For this review, take the finished solid that the model builds, in its own axes (mm). A direction names the side the tool comes from. Coordinates: 2 decimals unless noted, no trailing zeros. Loops run counter-clockwise (first coordinate to the right, second up) from the corner with the lowest first, then second, coordinate; pieces in that order, holes last. Notation, with made-up numbers: M 67,30 L 98,30 A23 ccw 98,41 Z; hole C -17.75,-13.5 d7. An arc over 180 degrees is marked long. Answer as a JSON object with one key per item and string values. Group by question number.
Item 1: Tool access review of faces 1 (the face through (0, 3, 1.85)), 2 (the face through (0, 3, -1.85)), 3 (the face through (-1.595, 3.161, -0.938)), 4 (the face through (-0.05, 6, -2.04)): name each direction out of +Z, -Z, +X, -X, +Y, -Y from which nothing blocks a thin tool from reaching the whole face with its end or side.
Item 2: Add section D-D (y = 6.5). State the section outline as (x, z) points.
Item 3: Wall thickness on L1, parallel to Y at x = -2, z = -2; L2, parallel to Z at x = 0.75, y = 3.5: over which ranges is each line inside the solid? List them lowest first. Write a range as from..to.
Item 4: Add section B-B (x = -0.5). State the section outline as (y, z) points.
Item 5: Insertion check: pin 1 (2 mm diameter, centred on x = 1.5, y = 4.5, fed in from -Z); pin 2 (2.5 mm diameter, centred on x = 0, y = 4, fed in from +Z). Each pin has a flat end and moves straight along its axis. Give the tip position at first contact, or say it passes through.
Item 6: Add section C-C (z = 1.25). State the section outline as (x, y) points.
Item 7: Add section A-A (y = 2.75). State the section outline as (x, z) points, then the cut area to 3 significant figures.
from build123d import *

# Parameters (mm, degrees)
BOSS_EXTRUDE1_DEPTH = 6
BOSS_EXTRUDE2_DEPTH = 1.2
CHAMFER1_SIZE       = 0.4


with BuildPart() as part:
    # Sketch1 → Boss-Extrude1 (new body)
    with BuildSketch(Plane(origin=(0, 0, 0), x_dir=(1, 0, 0), z_dir=(0, 1, 0))):
        Polygon((2.136195996, 0), (1.068097998, 1.85), (-1.068097998, 1.85), (-2.136195996, 0), (-1.068097998, -1.85), (1.068097998, -1.85), align=None)
    extrude(amount=BOSS_EXTRUDE1_DEPTH)

    # Sketch2 → Boss-Extrude2 (add)
    with BuildSketch(Plane(origin=(0, 6, 0), x_dir=(1, 0, 0), z_dir=(0, 1, 0))):
        Polygon((3.464101615, 0), (1.732050808, 3), (-1.732050808, 3), (-3.464101615, 0), (-1.732050808, -3), (1.732050808, -3), align=None)
    extrude(amount=BOSS_EXTRUDE2_DEPTH)

    # Chamfer1
    chamfer1_edges = [part.edges().sort_by_distance(p)[0] for p in [
        (0, 0, 1.85),
        (-1.602146997, 0, 0.925),
        (-1.602146997, 0, -0.925),
        (0, 0, -1.85),
        (1.602146997, 0, -0.925),
        (1.602146997, 0, 0.925),
    ]]
    chamfer(chamfer1_edges, length=CHAMFER1_SIZE)


solid = part.part
From the geometry:
{
 "1": {"face 1": "+Z, +X, -X, -Y", "face 2": "-Z, +X, -X, -Y", "face 3": "-Z, -X, -Y", "face 4": "-Y"},
 "2": {"outline": "M -3.46,0 L -1.73,-3 L 1.73,-3 L 3.46,0 L 1.73,3 L -1.73,3 Z"},
 "3": {"L1": "y = 6..7.2", "L2": "z = -1.85..1.85"},
 "4": {"outline": "M 0,-1.45 L 0.4,-1.85 L 6,-1.85 L 6,-3 L 7.2,-3 L 7.2,3 L 6,3 L 6,1.85 L 0.4,1.85 L 0,1.45 Z"},
 "5": {"pin 1": "stops at z = -1.85", "pin 2": "stops at z = 1.85"},
 "6": {"outline": "M -2.74,6 L -1.41,6 L -1.41,0.4 L -0.95,0 L 0.95,0 L 1.41,0.4 L 1.41,6 L 2.74,6 L 2.74,7.2 L -2.74,7.2 Z"},
 "7": {"outline": "M -2.14,0 L -1.07,-1.85 L 1.07,-1.85 L 2.14,0 L 1.07,1.85 L -1.07,1.85 Z", "area": "11.9 mm²"}
}
